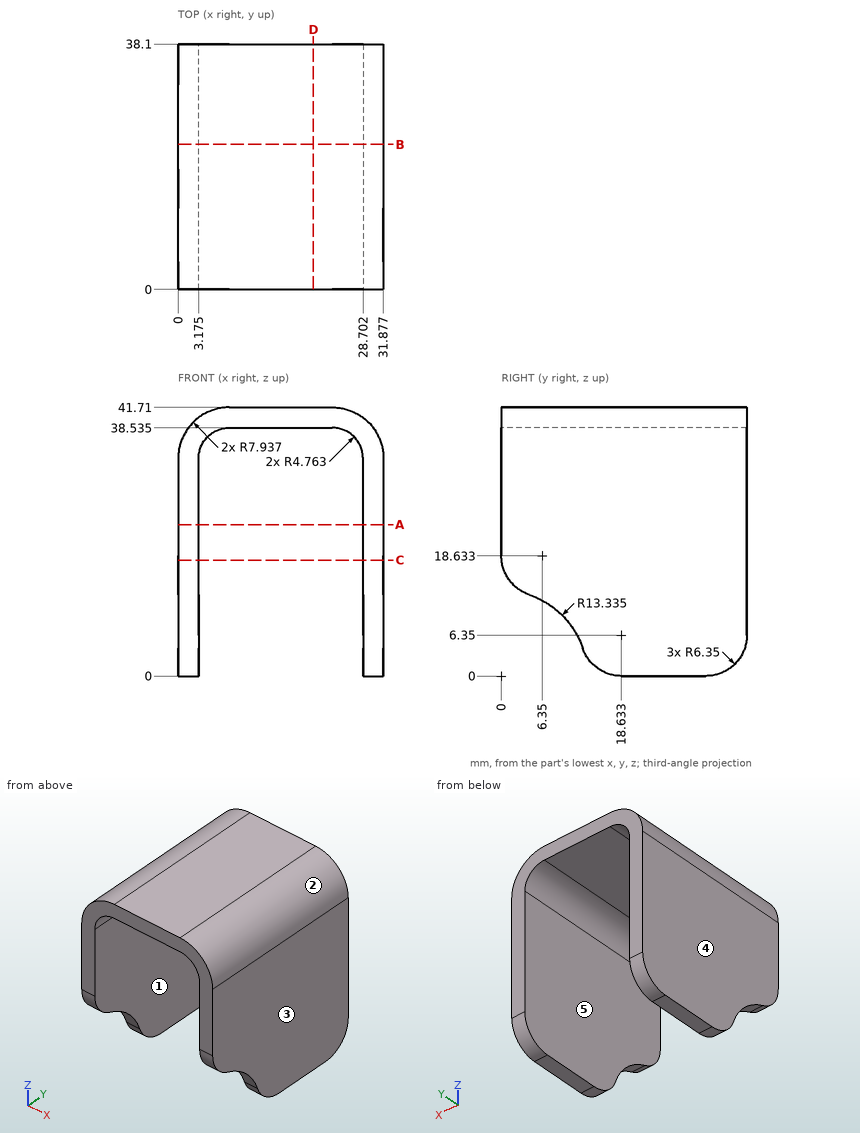
Can you work these out from the drawing? Everything is in mm from the part's minimum corner. A direction names the side the tool comes from. Round coordinates to 2 decimals unless told otherwise and drop trailing zeros. Loops run counter-clockwise (first coordinate to the right, second up) from the corner with the lowest first, then second, coordinate; pieces in that order, holes last.
1. If I drill on line 1 along X through (y, z) = (31, 32.5) (1 decimal); line 2 along Z through (x, y) = (21.5, 33.5) (1 decimal); line 3 along X through (y, z) = (24, 35.5) (1 decimal), over which ranges is the centre line in solid material (lowest first)?
Answer list:
line 1: x = 0 to 3.2, 28.7 to 31.9
line 2: z = 38.5 to 41.7
line 3: x = 0.2 to 3.5, 28.4 to 31.7
2. If we section it at B-B on y = 22.5: Write out the boundary of the cut face in (x, z) (1 decimal).
Answer list:
outline: (0, 0) - (3.2, 0) - (3.2, 33.8) arc R4.8 cw to (7.9, 38.5) - (23.9, 38.5) arc R4.8 cw to (28.7, 33.8) - (28.7, 0) - (31.9, 0) - (31.9, 33.8) arc R7.9 ccw to (23.9, 41.7) - (7.9, 41.7) arc R7.9 ccw to (0, 33.8) - close
3. Which directions (+Z, -Z, +X, -X, +Y, -Y) give clear straight access to the entire face, cutting with the end or side of a thin tool? Please do the marked faces 1 and 2.
Answer list:
face 1: -Z, +Y, -Y
face 2: +Z, +X, +Y, -Y
4. If we section it at A-A on z = 23.5: Write out the boundary of the cut face in (x, y) (1 decimal), plus the area to 3 significant figures.
Answer list:
outline: (0, 0) - (3.2, 0) - (3.2, 38.1) - (0, 38.1) - close; (28.7, 0) - (31.9, 0) - (31.9, 38.1) - (28.7, 38.1) - close
area: 242 mm2
5. We'd pull the mould along X, two halves only. Please class the marked faces 3, 4 and 5: +X half, -X half, draft (parallel to the pull), parting line (faces both ways), or undercut.
Answer list:
face 3: +X half
face 4: -X half
face 5: undercut
6. For P1, Ø1.5, axis at x = 6.5, y = 8, coming from the -Z side; P2, Ø10, axis at x = 17, y = 29, coming from the -Z side (1 decimal); P3, Ø6, axis at x = 23.5, y = 28, coming from the -Z side, each with a flat end and sliding along its axis, tell me the tip position at first contact or that it passes through.
Answer list:
P1: stops at z = 38
P2: stops at z = 38.5
P3: stops at z = 37.79
7. If we section it at D-D on x = 21: Write out the boundary of the cut face in (y, z) (1 decimal).
Answer list:
outline: (0, 38.5) - (38.1, 38.5) - (38.1, 41.7) - (0, 41.7) - close
